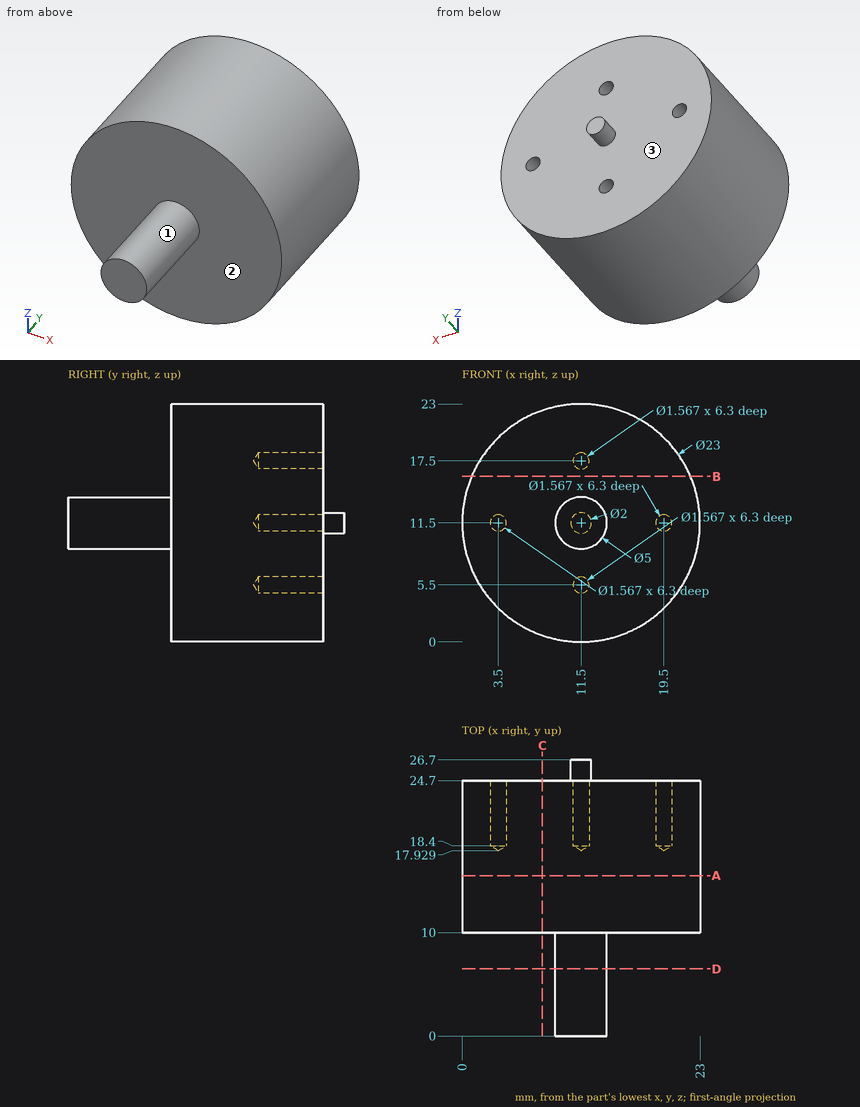
Drawing for the job (mm, zero at the part's lowest x, y, z). Round coordinates to 2 decimals unless told otherwise and drop trailing zeros. Loops run counter-clockwise (first coordinate to the right, second up) from the corner with the lowest first, then second, coordinate; pieces in that order, holes last. Notation, with made-up numbers: (-16.75, -36.75) - (34.25, -36.75) arc R10 ccw to (34.25, -23.75) - close; hole circle Ø2 at (68.5, -3). An arc over 180 degrees is marked (long way). Write each question's results on one line, items separated by ' | '.
(1) Saw through at D-D, the plane y = 6.5. List the corners of the cut face in (x, z).
Answer below:
outline: circle Ø5 at (11.5, 11.5)
(2) Saw through at C-C, the plane x = 7.75. List the corners of the cut face in (y, z), then the cut area to 3 significant figures.
Answer below:
outline: (10, 0.63) - (24.7, 0.63) - (24.7, 22.37) - (10, 22.37) - close | area: 320 mm^2
(3) Mould opens along Y. For the marked faces 1, 2 and 3 say: released by +Y, released by -Y, zero draft, split by the parting line, or undercut.
Answer below:
face 1: zero draft | face 2: released by -Y | face 3: released by +Y
(4) Saw through at B-B, the plane z = 16. List the corners of the cut face in (x, y).
Answer below:
outline: (0.92, 10) - (22.08, 10) - (22.08, 24.7) - (0.92, 24.7) - close
(5) Saw through at A-A, the plane y = 15.5. List the corners of the cut face in (x, z).
Answer below:
outline: circle Ø23 at (11.5, 11.5)
(6) Pin check, flat tips, straight feed: pin 1 (11.5 mm diameter, centred on x = 10, z = 16.5, fed in from +Y); pin 2 (6 mm diameter, centred on y = 7.5, z = 13.5, fed in from +X) (3 decimals); pin 3 (1.4 mm diameter, centred on x = 3.5, z = 11.5, fed in from +Y); pin 4 (0.9 mm diameter, centred on x = 11.5, z = 5.5, fed in from -Y). Stop position of each tip, or through.
Answer below:
pin 1: stops at y = 26.7 | pin 2: stops at x = 22.995 | pin 3: stops at y = 18.35 | pin 4: stops at y = 10
(7) Wall check: L1, parallel to X at y = 23, z = 11.5; L2, parallel to Z at x = 11.5, y = 22.5; L3, parallel to Y at x = 11.25, z = 10.25. Give the ranges that are in metal, low to high.
Answer below:
L1: x = 0 to 2.72, 4.28 to 18.72, 20.28 to 23 | L2: z = 0 to 4.72, 6.28 to 16.72, 18.28 to 23 | L3: y = 0 to 24.7
